Geometry: see drawing. Coordinates: mm, zero at the bounding-box minimum. Give positions to 0.01 mm unless a question says otherwise; leave off trailing zeros. Write each loop counter-clockwise with the first axis right and the second up, starting at its lowest first coordinate (ties: lowest second). Pieces come first, ordered by that corner, then holes. Notation, with made-up numbers: (10.5, 67) -> (54.5, 67) arc R31 cw to (54.5, 99) -> close; hole circle Ø8 at (51, 48.25). An arc over 180 degrees is marked (long way). Write item = value, one per line.
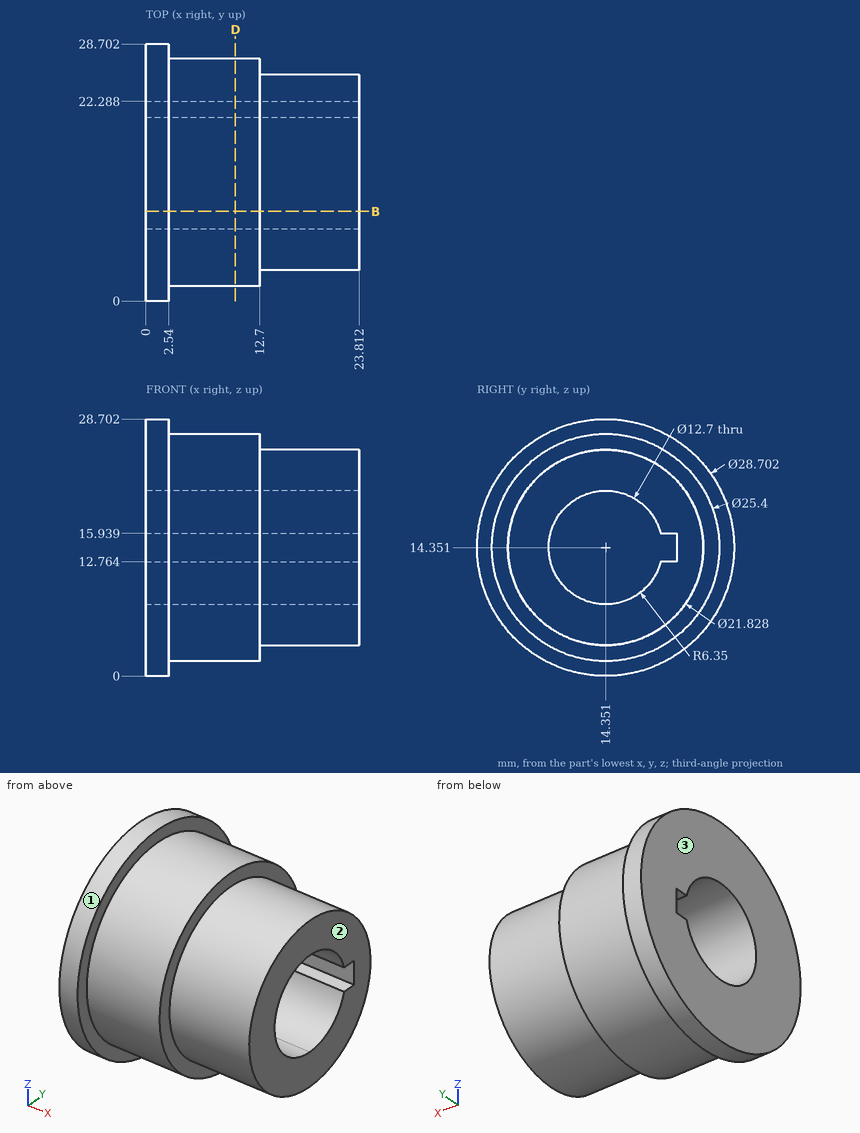
(1) First-contact query: pin 1 (1.4 mm diameter, centred on x = 8, y = 21.5, fed in from +Z); pin 2 (4 mm diameter, centred on x = 3.5, z = 5, fed in from +Y) (1 decimal); pin 3 (12.5 mm diameter, centred on y = 8.5, z = 14, fed in from +X); pin 4 (1 mm diameter, centred on x = 7, z = 7, fed in from +Y) (1 decimal). Flat tips, straight axial feed; report the tip coordinate or a pass-through.
Values follow:
pin_1 = 25.29
pin_2 = 26.5
pin_3 = 23.81
pin_4 = 25
(2) Pull-direction query (X, two-part tool) for the marked faces 1, 2 and 3; classes: pulls with the +X half, pulls with the -X half, needs draft (parallel to the pull), parting line crosses it, or undercut.
Values follow:
face_1 = needs draft
face_2 = pulls with the +X half
face_3 = pulls with the -X half
(3) Material intervals for line 1 (X direction, y = 25.5, z = 9); line 2 (Y direction, x = 21, z = 15.25) (1 decimal); line 3 (Y direction, x = 12.75, z = 14.75) (1 decimal), sorted ascending.
Values follow:
line_1 = 0 to 12.7
line_2 = 3.5 to 8.1, 22.3 to 25.2
line_3 = 3.4 to 8, 22.3 to 25.3
(4) Section query D-D (x = 10). Return loops of the section in (y, z), plus the area to 3 significant figures.
Values follow:
outline = circle Ø25.4 at (14.35, 14.35); hole (20.5, 12.76) -> (22.29, 12.76) -> (22.29, 15.94) -> (20.5, 15.94) arc R6.35 ccw (long way) to start
area = 375 mm2
(5) Section query B-B (y = 10). Return loops of the section in (x, z) (1 decimal).
Values follow:
outline = (0, 0.7) -> (2.5, 0.7) -> (2.5, 2.4) -> (12.7, 2.4) -> (12.7, 4.3) -> (23.8, 4.3) -> (23.8, 9.7) -> (0, 9.7) -> close; (0, 19) -> (23.8, 19) -> (23.8, 24.4) -> (12.7, 24.4) -> (12.7, 26.3) -> (2.5, 26.3) -> (2.5, 28) -> (0, 28) -> close
